Build history of the part. All positions in model axes, mm. Face numbers are marked on the shaded views. A direction names the side the tool comes from. Give positions to 0.01 mm unless a question says otherwise; leave off trailing zeros. Write each loop counter-clockwise with the first axis right and the second up, starting at its lowest first coordinate (ties: lowest second). Pieces come first, ordered by that corner, then holes. Notation, with made-up numbers: (-16.5, -32) -> (30.5, -32) arc R8 ccw to (30.5, -28) -> close; hole circle Ø9 at (45.25, -39.75). An arc over 180 degrees is marked (long way). One line per question, with ' | ' between items. Start each with the question number.
(1) Band-saw the part on B-B, the plane y = 0.5. Give the cut face in (x, z).
(2) Band-saw the part on D-D, the plane x = 8.75. Give the cut face in (y, z), and give its area (3 significant figures).
(3) Band-saw the part on C-C, the plane x = 0. Count the separate pieces of the cut face and the enclosed holes in it, and give its area (3 significant figures).
(4) Pin check, flat tips, straight feed: P1, Ø0.5, axis at y = 1.5, z = -11.5, coming from the +X side; P2, Ø0.9, axis at y = 2, z = -29.5, coming from the +X side; P3, Ø0.5, axis at y = 1.5, z = -14.5, coming from the -X side. Stop position of each tip, or through.
(5) Pull direction Z, two halves, no side cores. Call the marked faces 1, 2 and 3: released by +Z, released by -Z, zero draft, split by the parting line, or undercut.
(6) Tool access for the marked faces 4, 5 and 6: list every direction of +Z, -Z, +X, -X, +Y, -Y with a clear straight run to the whole face (end or side of a thin tool).
(7) Drill centre lines: probe 1 along Z at (x, y) = (-5.75, -3.25); probe 2 along Z at (x, y) = (0, 1.1); probe 3 along X at (y, z) = (0.5, -25). Where is each one in solid material? Low to high. Write a range as from..to.
Autodesk Inventor part; units mm, degrees
ref_plane "YZ Plane" through (0, 0, 0) normal (1, 0, 0) x (0, 1, 0)
ref_plane "XZ Plane" through (0, 0, 0) normal (0, 1, 0) x (-1, 0, 0)
ref_plane "XY Plane" through (0, 0, 0) normal (0, 0, 1) x (1, 0, 0)
sketch "Sketch15" plane through (0, 0, 0) normal (0, 1, 0) x (-1, 0, 0)
  circle A0 centre (0, 0) radius 2.75
  circle A1 centre (0, 0) radius 7.5
  line L0 (0, 0) -> (0, -28)
  line L1 (0, -33) -> (0, -23) construction
  line L2 (2.75, -33) -> (2.75, -23)
  line L3 (-2.75, -23) -> (-2.75, -33)
  arc A2 (-2.75, -33) -> (2.75, -33) centre (0, -33) ccw
  arc A3 (2.75, -23) -> (-2.75, -23) centre (0, -23) ccw
  line L4 (0, -43) -> (0, -13) construction
  line L5 (0, 0) -> (0, -14)
  line L6 (-10, -15.5) -> (10, -15.5)
  line L7 (10, -15.5) -> (10, -10.5)
  line L8 (10, -10.5) -> (-10, -10.5)
  line L9 (-10, -10.5) -> (-10, -15.5)
  line L10 (-10, -15.5) -> (10, -10.5) construction
  line L11 (10, -15.5) -> (-10, -10.5) construction
  line L12 (7.4616, 0.7577) -> (10, -10.5)
  line L13 (-7.4616, 0.7577) -> (-10, -10.5)
  line L14 (0, -35.75) -> (0, -20.25) construction
  line L15 (10, -35.75) -> (10, -20.25)
  line L16 (-10, -20.25) -> (-10, -35.75)
  arc A4 (-10, -35.75) -> (10, -35.75) centre (0, -35.75) ccw
  arc A5 (10, -20.25) -> (-10, -20.25) centre (0, -20.25) ccw
  line L17 (10, -15.5) -> (10, -20.25)
  line L18 (-10, -15.5) -> (-10, -20.25)
  line L19 (0, 0) -> (0, 25)
  circle A6 centre (0, 25) radius 2.75
  circle A7 centre (0, 25) radius 5
  line L20 (0, 25) -> (5, 25)
  line L21 (0, 25) -> (-5, 25)
  line L22 (5, 25) -> (7.4616, 0.7577)
  line L23 (-5, 25) -> (-7.4616, 0.7577)
  point P0 (-8.7999, -15.5)
  point P1 (8.7999, -15.5)
  dimension "d102" = 5.5
  dimension "d103" = 15
  dimension "d104" = 28
  dimension "d105" = 5
  dimension "d106" = 5.5
  dimension "d107" = 15
  dimension "d109" = 14
  dimension "d110" = 20
  dimension "d111" = 5
  dimension "d112" = 20
  dimension "d133" = 25
  dimension "d134" = 5.5
  dimension "d135" = 10
extrude "Extrusion14" add sketch "Sketch15" along normal blind 1 contours A0 L19 A1 L0 | A0 L0 A1 L19 | L19 A7 L22 A1 | A1 L23 A7 L19 | L0 A5 L8 L13 A1 | A1 L12 L8 A5 L0 | A7 L21 A6 L19 | L19 A6 L20 A7 | A5 L8 L0 | L0 L8 A5 | L7 L6 A5 L8 | L20 A6 L21 A7 | L8 A5 L6 L9 | L8 A5 L6 L0 | L0 L6 A5 L8 | L17 A5 L6 | L6 A5 L18 | A5 L15 A4 L16 L6
sketch "Sketch16" plane through (0, 1, 0) normal (0, 1, 0) x (1, 0, 0)
  circle A0 centre (0, 0) radius 2.75
  circle A1 centre (0, 0) radius 2.75
  line L0 (-2.75, 23) -> (-2.75, 33)
  line L1 (-2.75, 28) -> (0, 28)
  line L2 (0, 33) -> (0, 23) construction
  line L3 (-2.75, 33) -> (-2.75, 23)
  line L4 (2.75, 23) -> (2.75, 33)
  arc A2 (2.75, 33) -> (-2.75, 33) centre (0, 33) ccw
  arc A3 (-2.75, 23) -> (2.75, 23) centre (0, 23) ccw
  line L5 (0, 33) -> (0, 23) construction
  line L6 (-4, 33) -> (-4, 23)
  line L7 (4, 23) -> (4, 33)
  arc A4 (4, 33) -> (-4, 33) centre (0, 33) ccw
  arc A5 (-4, 23) -> (4, 23) centre (0, 23) ccw
  circle A6 centre (0, -25) radius 2.75
  circle A7 centre (0, -25) radius 2.75
  circle A8 centre (0, -25) radius 5
  circle A9 centre (0, 0) radius 5
  point P0 (-7.4616, -0.7577)
  point P1 (-2.75, 33)
  dimension "d115" = 5
  dimension "d116" = 5.5
  dimension "d117" = 5
  dimension "d118" = 8
  dimension "d136" = 5.5
  dimension "d137" = 10
  dimension "d138" = 10
extrude "Extrusion15" add sketch "Sketch16" along normal blind 2
sketch "Sketch17" plane through (0, 1, 0) normal (0, 1, 0) x (1, 0, 0)
  line L0 (0, 0) -> (0, 13)
  line L1 (7.5, 17) -> (-7.5, 17)
  line L2 (-7.5, 17) -> (-7.5, 9)
  line L3 (-7.5, 9) -> (7.5, 9)
  line L4 (7.5, 9) -> (7.5, 17)
  line L5 (7.5, 17) -> (-7.5, 9) construction
  line L6 (-7.5, 17) -> (7.5, 9) construction
  dimension "d121" = 13
  dimension "d129" = 15
  dimension "d130" = 8
extrude "Extrusion16" add sketch "Sketch17" along normal blind 2
fillet "Fillet7" radius 1 4 edges at (-7.5, 2, -9) (-7.5, 2, -17) (7.5, 2, -9) (7.5, 2, -17)
fillet "Fillet8" radius 1 8 edges at (7.2071, 3, -9.2929) (7.5, 3, -13) (7.2071, 3, -16.7071) (0, 3, -17) (-7.2071, 3, -16.7071) (-7.5, 3, -13) (-7.2071, 3, -9.2929) (0, 3, -9)
sketch "Sketch18" plane through (0, 0, 0) normal (0, -1, 0) x (1, 0, 0)
  arc A0 (2.75, -23) -> (-2.75, -23) centre (0, -23) ccw
  arc A1 (-2.75, -33) -> (2.75, -33) centre (0, -33) ccw
  line L0 (0, -23) -> (0, -33) construction
  line L1 (-7.5, -23) -> (-7.5, -33)
  line L2 (7.5, -33) -> (7.5, -23)
  arc A2 (7.5, -23) -> (-7.5, -23) centre (0, -23) ccw
  arc A3 (-7.5, -33) -> (7.5, -33) centre (0, -33) ccw
  circle A4 centre (0, 0) radius 7.5
  circle A5 centre (0, 25) radius 2.75
  circle A6 centre (0, 25) radius 6
  point P0 (0, -28)
  dimension "d139" = 15
  dimension "d143" = 15
  dimension "d144" = 12
move faces "Move1" translate (0, -5, 0) faces at (-7.5833, 0, -23.0833)
extrude "Extrusion17" cut sketch "Sketch18" along normal blind 10
sketch "Sketch19" plane through (0, -5, -35.75) normal (0, -1, 0) x (1, 0, 0)
  circle A0 centre (0, 60.75) radius 2.75
  circle A1 centre (0, 60.75) radius 15
  point P0 (0, 35.75)
  dimension "d147" = 30
extrude "Extrusion18" cut sketch "Sketch19" against normal through all
fillet "Fillet9" radius 2 4 edges at (0, 0, -15.5) (-7.5, 0, -28) (0, 0, -40.5) (7.5, 0, -28)
properties part number "Belt_Restraint"
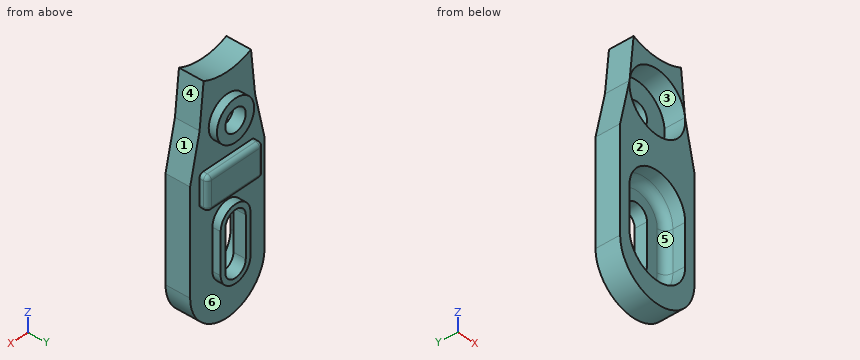
Results:
1) outline: (-10, -35.75) arc R10 ccw to (10, -35.75) -> (10, -10.5) -> (7.46, 0.76) -> (6.38, 11.42) arc R15 cw to (-6.38, 11.42) -> (-7.46, 0.76) -> (-10, -10.5) -> close; hole (-2.75, -33) arc R2.75 ccw to (2.75, -33) -> (2.75, -23) arc R2.75 ccw to (-2.75, -23) -> close; hole circle Ø5.5 at (0, 0)
2) outline: (-5, -40.59) -> (1, -40.59) -> (1, -4.96) -> (-5, -4.96) -> close | area: 214 mm²
3) separate pieces: 3 | enclosed holes: 0 | area: 145 mm²
4) P1: stops at x = 7.5 | P2: stops at x = 4 | P3: stops at x = -7.5
5) face 1: released by +Z | face 2: zero draft | face 3: undercut
6) face 4: +Z, +X, +Y, -Y | face 5: -Y | face 6: +Y
7) probe 1: z = -43.93..-37.82, -18.18..-4.82, 4.82..11.15 | probe 2: z = -37..-35.75, -20.25..-19, -17..-9, -5..-2.75, 2.75..5 | probe 3: x = -10..-2.75, 2.75..10
